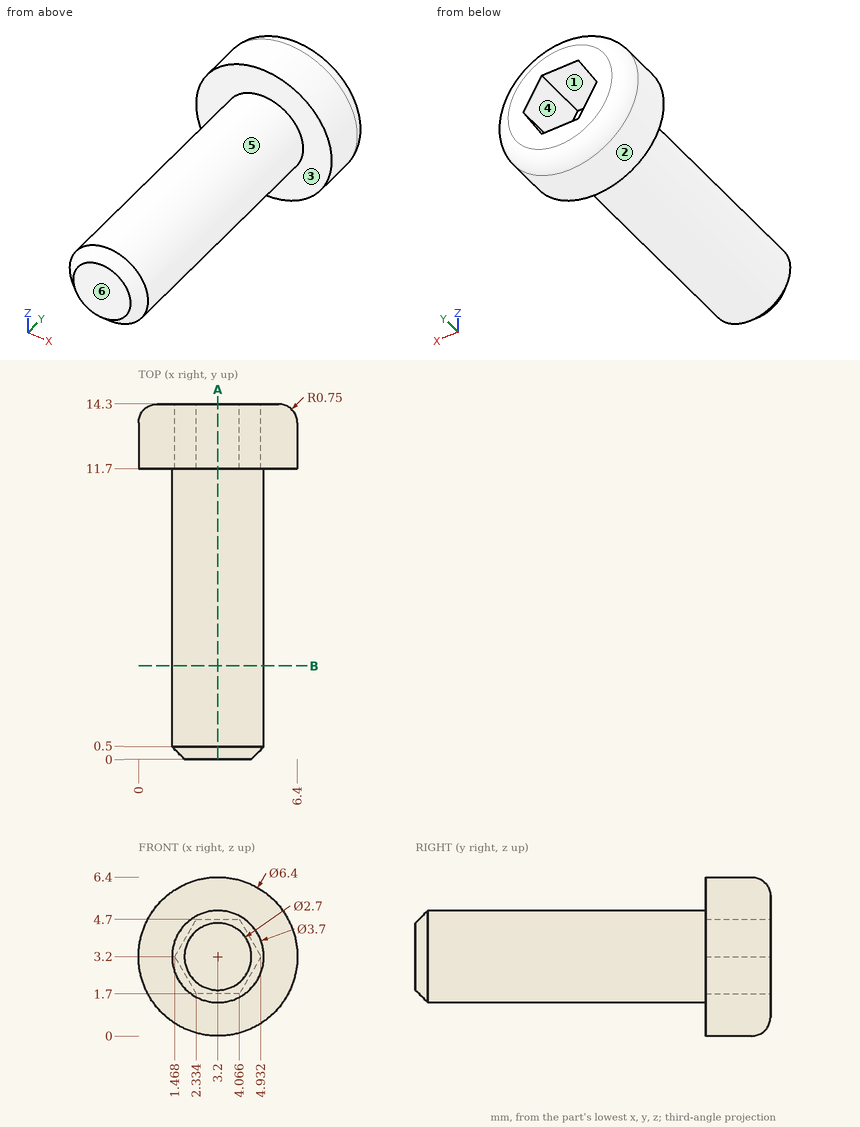
The figure shows three views and two pictorial views of one solid part (mm, origin at its lowest corner). Answer the questions. A direction names the side the tool comes from. Round coordinates to 2 decimals unless told otherwise and drop trailing zeros. Order: outer loops, then holes, each group sorted by start corner. A loop starts at its lowest first (then second) coordinate and runs counter-clockwise, first axis right, second up. Notation, with made-up numbers: M 57,9 L 92,9 A28 ccw 92,45 Z; hole C 64,76 d10. An arc over 180 degrees is marked long. Answer in a Markdown table with one row per item. Add a question column.
1) The part is cut by section A-A on x = 3.2. Determine the outline of the cut face in (y, z).
2) Consider line 1 along Y through (x, z) = (3, 3.5); line 2 along Y through (x, z) = (1, 2); line 3 along X through (y, z) = (7.75, 3.25). Determine where each line is inside the solid, lowest interval first. Write a range as from..to.
3) A flat-ended cylindrical pin translates along its axis: pin 1 Ø3 at (y, z) = (7.5, 1) entering from +X. Find the tip coordinate at first contact, or state that the pin passes through.
4) Which of the six approach directions +Z, -Z, +X, -X, +Y, -Y give full straight-line access (tool end or side, diameter ignored) to the marked faces 1, 2 and 3?
5) Determine the mould class of the marked faces 4, 5 and 6 for opening direction Z: pulls with the +Z half, pulls with the -Z half, needs draft (parallel to the pull), parting line crosses it, or undercut.
6) The part is cut by section B-B on y = 3.75. Determine the outline of the cut face in (x, z).
Findings below:
| question | item | result |
|---|---|---|
| 1 | outline | M 0,1.85 L 0.5,1.35 L 11.7,1.35 L 11.7,0 L 13.55,0 A0.75 ccw 14.3,0.75 L 14.3,1.7 L 11.7,1.7 L 11.7,4.7 L 14.3,4.7 L 14.3,5.65 A0.75 ccw 13.55,6.4 L 11.7,6.4 L 11.7,5.05 L 0.5,5.05 L 0,4.55 Z |
| 2 | line 1 | y = 0..11.7 |
| 2 | line 2 | y = 11.7..14.3 |
| 2 | line 3 | x = 1.35..5.05 |
| 3 | pin 1 | stops at x = 4.91 |
| 4 | face 1 | +Y |
| 4 | face 2 | +Y, -Y |
| 4 | face 3 | -Y |
| 5 | face 4 | undercut |
| 5 | face 5 | parting line crosses it |
| 5 | face 6 | needs draft |
| 6 | outline | C 3.2,3.2 d3.7 |
